```python
from build123d import *

# Parameters (mm, degrees)
SKETCH1_W           = 4.06
SKETCH1_H           = 5.33
BOSS_EXTRUDE1_DEPTH = 6.35
SKETCH2_R           = 1.55
BOSS_EXTRUDE2_DEPTH = 2.8702
FILLET2_R           = 1.55
SKETCH4_W           = 3.493828458
SKETCH4_H           = 0.340679683
CUT_EXTRUDE1_DEPTH  = 9.53535588
SKETCH6_W           = 0.6
SKETCH6_H           = 0.632779055
SKETCH6_H_2         = 0.632779056
BOSS_EXTRUDE5_DEPTH = 3.81


with BuildPart() as part:
    # Sketch1 → Boss-Extrude1 (new body)
    with BuildSketch(Plane(origin=(0, 0, 0), x_dir=(1, 0, 0), z_dir=(0, 1, 0))):
        Rectangle(SKETCH1_W, SKETCH1_H)
    extrude(amount=BOSS_EXTRUDE1_DEPTH)

    # Sketch2 → Boss-Extrude2 (add)
    with BuildSketch(Plane.XY.offset(2.665)):
        with Locations(Location((0, 3.05, 0), (0, 0, 180))):
            Circle(SKETCH2_R)
    extrude(amount=BOSS_EXTRUDE2_DEPTH)

    # Fillet2
    fillet2_edges = [part.edges().sort_by_distance(p)[0] for p in [
        (1.55, 3.05, 5.5352),
    ]]
    fillet(fillet2_edges, radius=FILLET2_R)

    # Sketch4 → Cut-Extrude1 (cut, through all)
    with BuildSketch(Plane.XY.offset(2.665)):
        with Locations((-0.015737966, 0.170339842)):
            Rectangle(SKETCH4_W, SKETCH4_H)
    extrude(amount=-CUT_EXTRUDE1_DEPTH, mode=Mode.SUBTRACT)

    # Sketch6 → Boss-Extrude5 (add)
    with BuildSketch(Plane.XZ.offset(-0.340679683)):
        with Locations((-1.278193782, -1.380000213)):
            Rectangle(SKETCH6_W, SKETCH6_H)
        with Locations((1.261806218, -1.395)):
            Rectangle(SKETCH6_W, SKETCH6_H_2)
    extrude(amount=BOSS_EXTRUDE5_DEPTH)


solid = part.part
```
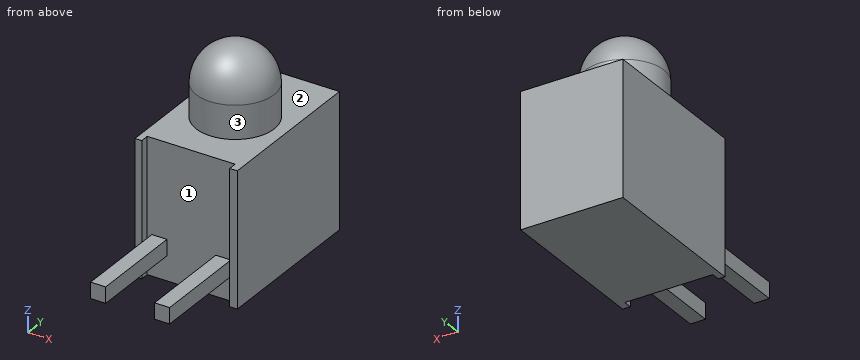
The model under review builds one solid part; all positions refer to its coordinate system, in mm. Face numbers are marked on the shaded views. Coordinates: 2 decimals unless noted, no trailing zeros. Order: outer loops, then holes, each group sorted by start corner. A loop starts at its lowest first (then second) coordinate and runs counter-clockwise, first axis right, second up. Notation, with made-up numbers: (-6.5, 1.25) -> (31.5, 1.25) arc R31 cw to (31.5, 34.25) -> close; hole circle Ø9 at (50.5, 45.5). An arc over 180 degrees is marked (long way). Answer in a Markdown table with one row per item. Add a question column.
Item 1: Clearance check with flat-ended pins moving along their axes: pin 1 (0.5 mm diameter, centred on x = -1, y = -1.5, fed in from +Z); pin 2 (0.5 mm diameter, centred on y = -1, z = -1.5, fed in from +X); pin 3 (0.7 mm diameter, centred on x = 1, y = -1, fed in from -Z). State where each tip first meets the part, or that it passes through.
Item 2: We need section D-D on x = -1.1. Write out the cut boundary in (y, z) (3 decimals).
Item 3: We need section B-B on x = 0. Write out the cut boundary in (y, z) (3 decimals), plus the area to 3 significant figures.
Item 4: To check wall thickness, follow probe 1 along Z at (x, y) = (1.35, -2); probe 2 along Z at (x, y) = (-0.8, 1.5) (3 decimals); probe 3 along Y at (x, z) = (-0.15, 0.25). State the ranges of each line that lie inside material, in increasing order.
Item 5: Mouldability with a two-part tool opening along X and no side actions: class the marked faces 1, 2 and 3 as +X half, -X half, draft (parallel to the pull), parting line (faces both ways), or undercut.
Item 6: We need section C-C on z = 1.75. Write out the cut boundary in (x, y), plus the area to 3 significant figures.
Item 7: We need section A-A on y = -0.25. Write out the cut boundary in (x, z).
Final values:
| question | item | result |
|---|---|---|
| 1 | pin 1 | stops at z = -1.06 |
| 1 | pin 2 | stops at x = 1.56 |
| 1 | pin 3 | stops at z = -1.71 |
| 2 | outline | (-3.469, -1.696) -> (0.341, -1.696) -> (0.341, -2.665) -> (6.35, -2.665) -> (6.35, 2.665) -> (4.142, 2.665) -> (4.142, 3.985) arc R1.092 ccw to (1.958, 3.985) -> (1.958, 2.665) -> (0.341, 2.665) -> (0.341, -1.064) -> (-3.469, -1.064) -> close |
| 3 | outline | (0.341, -2.665) -> (6.35, -2.665) -> (6.35, 2.665) -> (4.6, 2.665) -> (4.6, 3.985) arc R1.55 ccw to (1.5, 3.985) -> (1.5, 2.665) -> (0.341, 2.665) -> close |
| 3 | area | 39.9 mm2 |
| 4 | probe 1 | z = -1.71 to -1.08 |
| 4 | probe 2 | z = -2.665 to 2.665 |
| 4 | probe 3 | y = 0.34 to 6.35 |
| 5 | face 1 | undercut |
| 5 | face 2 | draft |
| 5 | face 3 | parting line |
| 6 | outline | (-2.03, 0) -> (-1.76, 0) -> (-1.76, 0.34) -> (1.73, 0.34) -> (1.73, 0) -> (2.03, 0) -> (2.03, 6.35) -> (-2.03, 6.35) -> close |
| 6 | area | 24.6 mm2 |
| 7 | outline | (-1.58, -1.7) -> (-0.98, -1.7) -> (-0.98, -1.06) -> (-1.58, -1.06) -> close; (0.96, -1.71) -> (1.56, -1.71) -> (1.56, -1.08) -> (0.96, -1.08) -> close |
